Source: three-view drawing plus pictorial views. Frame: mm from the lowest corner of the part. A direction names the side the tool comes from. Coordinates: 2 decimals unless noted, no trailing zeros. Order: outer loops, then holes, each group sorted by start corner. A loop starts at its lowest first (then second) coordinate and runs counter-clockwise, first axis right, second up. Notation, with made-up numbers: (77.5, -7.5) -> (122.5, -7.5) arc R22 cw to (122.5, 7.5) -> close; hole circle Ø4 at (69.5, -34). An arc over 180 degrees is marked (long way). Use one line per item in the form item = value. Start each with the question number.
1) Section query B-B on y = 30. Output: boundary loops of the cut face in (x, z) (3 decimals).
2) Draft query along Z for the marked faces 1, 2 and 3. Return one class per face: pulls with the +Z half, pulls with the -Z half, needs draft (parallel to the pull), parting line crosses it, or undercut.
3) Section query A-A on y = 2. Output: boundary loops of the cut face in (x, z).
4) Pin query (flat end, axial travel): pin 1 (6 mm diameter, centred on y = 30, z = 19, fed in from -X); pin 2 (2.5 mm diameter, centred on x = 3, y = 8.5, fed in from +Z); pin 3 (3 mm diameter, centred on x = 5, z = 17.5, fed in from -Y). Return the tip coordinate at first contact, or that it passes through.
5) Section query D-D on z = 50. Output: boundary loops of the cut face in (x, y) (3 decimals), then the cut area to 3 significant figures.
6) Access query for the marked faces 4 and 5. Directions: +Z, -Z, +X, -X, +Y, -Y. A direction counts if a zero-diameter tool reaches every point of the face in a straight line with its end or side. Return the directions, or none.
7) Section query C-C on x = 6.5. Output: boundary loops of the cut face in (y, z) (3 decimals).
8) Ray query, line 1 along Z through (x, y) = (3.5, 30) (3 decimals); line 2 along Z through (x, y) = (2.75, 12.5); line 3 along Y through (x, z) = (7.5, 18). Return the intervals inside material, ascending.
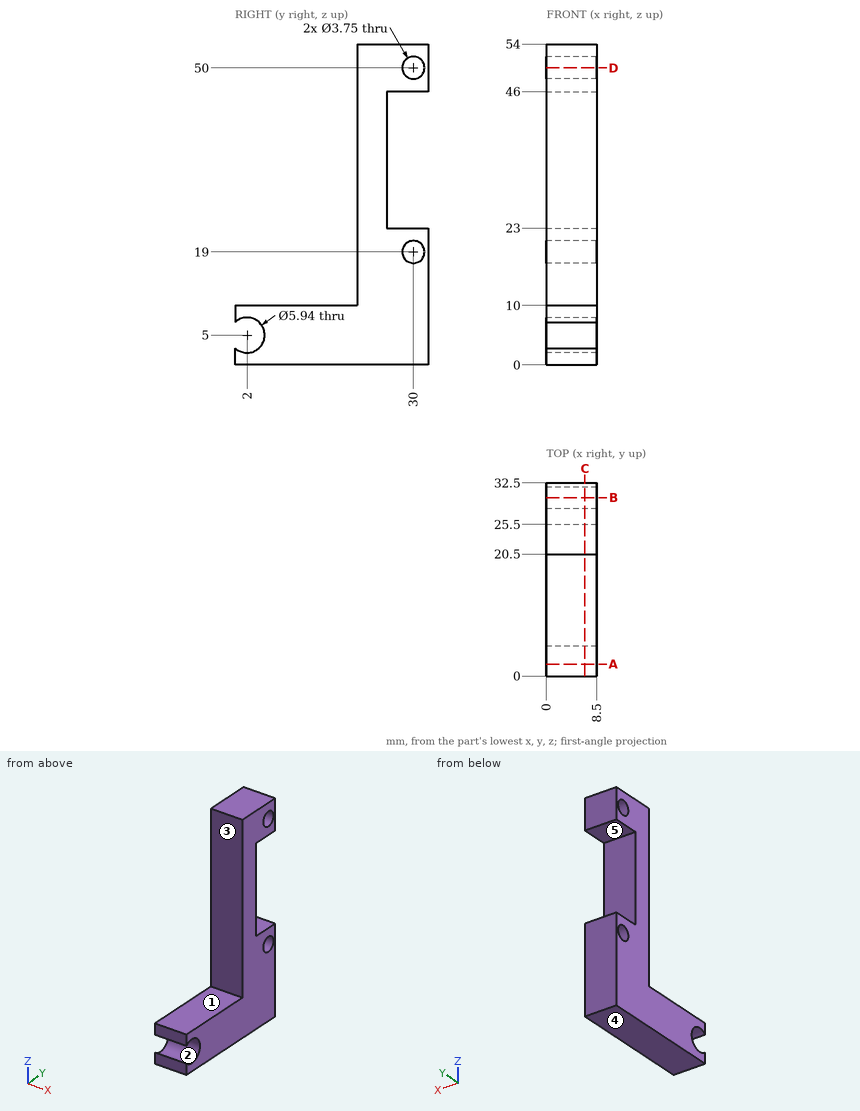
Answers below:
q1.outline = (0, 0) -> (8.5, 0) -> (8.5, 17.125) -> (0, 17.125) -> close; (0, 20.875) -> (8.5, 20.875) -> (8.5, 23) -> (0, 23) -> close; (0, 46) -> (8.5, 46) -> (8.5, 48.125) -> (0, 48.125) -> close; (0, 51.875) -> (8.5, 51.875) -> (8.5, 54) -> (0, 54) -> close
q2.face_1 = pulls with the +Z half
q2.face_2 = undercut
q2.face_3 = needs draft
q3.outline = (0, 0) -> (8.5, 0) -> (8.5, 2.03) -> (0, 2.03) -> close; (0, 7.97) -> (8.5, 7.97) -> (8.5, 10) -> (0, 10) -> close
q4.pin_1 = 0
q4.pin_2 = 10
q4.pin_3 = 20.5
q5.outline = (0, 20.5) -> (8.5, 20.5) -> (8.5, 28.125) -> (0, 28.125) -> close; (0, 31.875) -> (8.5, 31.875) -> (8.5, 32.5) -> (0, 32.5) -> close
q5.area = 70.1 mm^2
q6.face_4 = -Z, +X, -X, +Y, -Y
q6.face_5 = +X, -X, +Y
q7.outline = (0, 0) -> (32.5, 0) -> (32.5, 23) -> (25.5, 23) -> (25.5, 46) -> (32.5, 46) -> (32.5, 54) -> (20.5, 54) -> (20.5, 10) -> (0, 10) -> (0, 7.196) arc R2.97 cw (long way) to (0, 2.804) -> close; hole circle Ø3.75 at (30, 19); hole circle Ø3.75 at (30, 50)
q8.line_1 = 0 to 17.125, 20.875 to 23, 46 to 48.125, 51.875 to 54
q8.line_2 = 0 to 10
q8.line_3 = 20.5 to 28.41, 31.59 to 32.5
